Input: part model. Units: mm. Frame: model coordinates. Give positions to 0.01 mm unless a question says otherwise; leave off trailing zeros. Loops run counter-clockwise (first coordinate to the right, second up) from the corner with the lowest first, then second, coordinate; pieces in that order, holes last. Notation, with made-up numbers: (41.25, 22) - (68.25, 22) arc R16 cw to (68.25, 51) - close; hole circle Ø4 at (17, 79.5). An arc over 180 degrees is marked (long way). One line per item, written item: value.
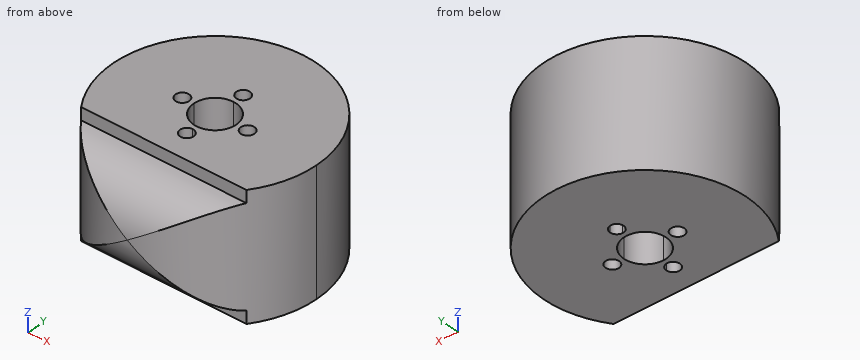
from build123d import *

# Parameters (mm, degrees)
F0_R     = 30.48
F0_R_2   = 2.032
F1_DEPTH = 37.338
F3_DEPTH = 39.58267
F4_DEPTH = 55.88364


with BuildPart() as f1:
    # F0 (on Top) → F1 (new body)
    with BuildSketch(Plane.XY):
        Circle(F0_R)
        with BuildLine():
            ThreePointArc((2.032, -9.779), (-1.4368409794, -11.2158409794), (0, -7.747))
            ThreePointArc((0, -7.747), (1.4368409794, -8.3421590206), (2.032, -9.779))
        make_face(mode=Mode.SUBTRACT)
        with Locations((-9.779, 0)):
            Circle(F0_R_2, mode=Mode.SUBTRACT)
        with BuildLine():
            ThreePointArc((0, 6.35), (4.4901280605, 4.4901280605), (6.35, 0))
            ThreePointArc((6.35, 0), (4.4901280605, -4.4901280605), (0, -6.35))
            ThreePointArc((0, -6.35), (-4.4901280605, -4.4901280605), (-6.35, 0))
            ThreePointArc((-6.35, 0), (-4.4901280605, 4.4901280605), (0, 6.35))
        make_face(mode=Mode.SUBTRACT)
        with BuildLine():
            ThreePointArc((11.811, 0), (9.779, -2.032), (7.747, 0))
            ThreePointArc((7.747, 0), (9.779, 2.032), (11.811, 0))
        make_face(mode=Mode.SUBTRACT)
        with BuildLine():
            ThreePointArc((2.032, 9.779), (1.4368409794, 8.3421590206), (0, 7.747))
            ThreePointArc((0, 7.747), (-1.4368409794, 11.2158409794), (2.032, 9.779))
        make_face(mode=Mode.SUBTRACT)
    extrude(amount=F1_DEPTH)

    # F2 (on Right) → F3 (cut)
    with BuildSketch(Plane.YZ):
        with BuildLine():
            Line((-30.48, 37.3969972134), (-30.48, 18.6984986067))
            ThreePointArc((-30.48, 18.6984986067), (-26.8779716111, 28.5202881076), (-17.78, 33.6844986067))
            Line((-17.78, 33.6844986067), (-17.78, 37.3969972134))
            Line((-17.78, 37.3969972134), (-30.48, 37.3969972134))
        make_face()
        with BuildLine():
            Line((-30.48, 0), (-17.78, 0))
            Line((-17.78, 0), (-17.78, 3.7124986067))
            ThreePointArc((-17.78, 3.7124986067), (-26.8779716111, 8.8767091058), (-30.48, 18.6984986067))
            Line((-30.48, 18.6984986067), (-30.48, 0))
        make_face()
    extrude(amount=-F3_DEPTH, mode=Mode.SUBTRACT)

    # F2 (on Right) → F4 (cut)
    with BuildSketch(Plane.YZ):
        with BuildLine():
            Line((-30.48, 37.3969972134), (-30.48, 18.6984986067))
            ThreePointArc((-30.48, 18.6984986067), (-26.8779716111, 28.5202881076), (-17.78, 33.6844986067))
            Line((-17.78, 33.6844986067), (-17.78, 37.3969972134))
            Line((-17.78, 37.3969972134), (-30.48, 37.3969972134))
        make_face()
        with BuildLine():
            Line((-30.48, 0), (-17.78, 0))
            Line((-17.78, 0), (-17.78, 3.7124986067))
            ThreePointArc((-17.78, 3.7124986067), (-26.8779716111, 8.8767091058), (-30.48, 18.6984986067))
            Line((-30.48, 18.6984986067), (-30.48, 0))
        make_face()
    extrude(amount=F4_DEPTH, mode=Mode.SUBTRACT)


solid = f1.part
Item 1: Material intervals for L1, parallel to Y at x = 0.5, z = 20.5; L2, parallel to X at y = -1, z = 9; L3, parallel to X at y = 4, z = 8.5, sorted ascending.
Verdict:
L1: y = -30.37 to -11.75, -7.81 to -6.33, 6.33 to 7.81, 11.75 to 30.48
L2: x = -30.46 to -11.55, -8.01 to -6.27, 6.27 to 8.01, 11.55 to 30.46
L3: x = -30.22 to -4.93, 4.93 to 30.22
Item 2: Section D-D, the plane x = 4.5. Output: boundary loops of the cut face in (y, z).
Verdict:
outline: (-30.15, 15.53) arc R15.19 ccw to (-17.78, 3.71) - (-17.78, 0) - (-4.48, 0) - (-4.48, 37.34) - (-17.78, 37.34) - (-17.78, 33.68) arc R15.19 ccw to (-30.15, 21.87) - close; (4.48, 0) - (30.15, 0) - (30.15, 37.34) - (4.48, 37.34) - close
Item 3: Pin query (flat end, axial travel): P1, Ø2.5, axis at x = -9.779, y = 0, coming from the +Z side; P2, Ø5, axis at x = 3, z = 26.5, coming from the +Y side; P3, Ø5, axis at y = -13.5, z = 19.5, coming from the -X side; P4, Ø5, axis at y = -7.5, z = 12, coming from the -X side. Return the tip coordinate at first contact, or that it passes through.
Verdict:
P1: passes through
P2: stops at y = 30.48
P3: stops at x = -28.43
P4: stops at x = -30.07
Item 4: Section A-A, the plane x = -10.5. Output: boundary loops of the cut face in (y, z).
Verdict:
outline: (-28.61, 11.4) arc R15.19 ccw to (-17.78, 3.71) - (-17.78, 0) - (-1.9, 0) - (-1.9, 37.34) - (-17.78, 37.34) - (-17.78, 33.68) arc R15.19 ccw to (-28.61, 25.99) - close; (1.9, 0) - (28.61, 0) - (28.61, 37.34) - (1.9, 37.34) - close
Item 5: Section C-C, the plane y = 4.5. Output: boundary loops of the cut face in (x, z), and give its area (3 significant figures).
Verdict:
outline: (-30.15, 0) - (-4.48, 0) - (-4.48, 37.34) - (-30.15, 37.34) - close; (4.48, 0) - (30.15, 0) - (30.15, 37.34) - (4.48, 37.34) - close
area: 1,920 mm^2
Item 6: Section B-B, the plane z = 32.5. Output: boundary loops of the cut face in (x, y).
Verdict:
outline: (-21.47, -21.64) - (21.47, -21.64) arc R30.48 ccw (long way) to start; hole circle Ø4.06 at (-9.78, 0); hole circle Ø12.7 at (0, 0); hole circle Ø4.06 at (0, -9.78); hole circle Ø4.06 at (0, 9.78); hole circle Ø4.06 at (9.78, 0)
